Autodesk Inventor part; units mm, degrees
ref_plane "YZ Plane" through (0, 0, 0) normal (1, 0, 0) x (0, 1, 0)
ref_plane "XZ Plane" through (0, 0, 0) normal (0, 1, 0) x (-1, 0, 0)
ref_plane "XY Plane" through (0, 0, 0) normal (0, 0, 1) x (1, 0, 0)
sketch "Sketch1" plane through (0, 0, 0) normal (0, 1, 0) x (-1, 0, 0)
  line L0 (57.5, -173) -> (57.5, -173) construction
  line L1 (-57.5, -173) -> (-57.5, 0) construction
  line L2 (-57.5, 0) -> (57.5, 0)
  line L3 (57.5, 0) -> (57.5, -173) construction
  line L4 (80.5, 0) -> (-80.5, 0) construction
  line L5 (0, -207.6) -> (0, 34.6) construction
  line L6 (57.5, -173) -> (-57.5, -173)
  line L7 (-57.5, -173) -> (-57.5, -173) construction
  line L8 (57.5, 0) -> (-55.1767, 0)
  line L9 (57.5, -40) -> (-57.5, -40) construction
  line L10 (-57.5, -40) -> (-57.5, 0)
  line L11 (-57.5, 0) -> (57.5, 0)
  line L12 (57.5, 0) -> (57.5, -40)
  line L13 (-57.5, -173) -> (-57.5, -40)
  line L14 (57.5, -173) -> (57.5, -40)
  point P0 (0, 0)
  dimension "width" = 115
  dimension "Length" = 173
  dimension "d2" = 115
  dimension "d112" = 40
extrude "Base" add sketch "Sketch1" against normal blind 5
sketch "Sketch11" plane through (0, 0, 0) normal (0, 1, 0) x (1, 0, 0)
  line L0 (0, 207.6) -> (0, -34.6) construction
  line L1 (-57.5, 0) -> (57.5, 0) construction
  line L2 (57.5, 173) -> (-57.5, 173)
  line L3 (-50, 18) -> (50, 18) construction
  line L4 (50, 18) -> (50, 48) construction
  line L5 (50, 48) -> (-50, 48) construction
  line L6 (-50, 48) -> (-50, 18) construction
  point P0 (0, 0)
  point P1 (50, 168)
  point P2 (-50, 168)
  dimension "d91" = 18
  dimension "d92" = 50
  dimension "d93" = 5
  dimension "d94" = 50
  dimension "d113" = 30
hole "Mounting Holes" at (50, 0, -18) at (-50, 0, -18) at (50, 0, -168) at (-50, 0, -168) at (-50, 0, -48) at (50, 0, -48) direction (0, -1, 0) diameter 3.4 depth 6
fillet "Fillet1" radius 5 4 edges at (-57.5, -2.5, 0) (57.5, -2.5, -173) (-57.5, -2.5, -173) (57.5, -2.5, 0)
sketch "Sketch12" plane through (0, 0, 0) normal (0, 1, 0) x (1, 0, 0)
  line L0 (-6, 149) -> (43, 149) construction
  line L1 (43, 149) -> (43, 91) construction
  line L2 (43, 91) -> (-6, 91) construction
  line L3 (-6, 91) -> (-6, 149) construction
  line L4 (-57.5, 168) -> (-57.5, 5)
  line L5 (0, 207.6) -> (0, -34.6)
  line L6 (-52.5, 0) -> (52.5, 0)
  circle A0 centre (-50, 48) radius 1.7
  line L7 (52.5, 173) -> (-52.5, 173)
  circle A1 centre (50, 48) radius 1.7
  circle A2 centre (50, 168) radius 1.7
  point P0 (0, 0)
  point P1 (0, 0)
  point P2 (52.2987, 0)
  point P3 (-57.5, 40)
  point P4 (0, 0)
  dimension "d104" = 58
  dimension "d263" = 24
  dimension "d266" = 49
  dimension "d267" = 7
hole "RasPi Mounting Holes" at (-6, 0, -149) at (43, 0, -149) at (43, 0, -91) at (-6, 0, -91) direction (0, -1, 0) diameter 3.4 depth 6
sketch "Sketch15" plane through (0, 0, 0) normal (0, 1, 0) x (1, 0, 0)
  line L0 (-18, 149) -> (-18, 87.5) construction
  line L1 (-18, 87.5) -> (-50, 87.5) construction
  line L2 (-50, 87.5) -> (-50, 149) construction
  line L3 (-50, 149) -> (-18, 149) construction
  line L4 (-52.5, 0) -> (52.5, 0)
  circle A0 centre (43, 149) radius 1.7
  circle A1 centre (50, 48) radius 1.7
  circle A2 centre (-50, 48) radius 1.7
  point P0 (0, 0)
  point P1 (0, 0)
  dimension "d122" = 32
  dimension "d123" = 61.5
hole "LM2596 Mounting Holes" at (-18, 0, -149) at (-18, 0, -87.5) at (-50, 0, -87.5) at (-50, 0, -149) direction (0, -1, 0) diameter 3.4 depth 6
sketch "Sketch16" plane through (0, 0, 0) normal (0, 1, 0) x (1, 0, 0)
  line L0 (-7.5, 16.5) -> (7.5, 16.5) construction
  line L1 (7.5, 16.5) -> (7.5, 30) construction
  line L2 (7.5, 30) -> (-7.5, 30) construction
  line L3 (-7.5, 30) -> (-7.5, 16.5) construction
  line L4 (52.5, 173) -> (-52.5, 173)
  line L5 (-52.5, 0) -> (52.5, 0)
  point P0 (0, 0)
  point P1 (0, 30)
  point P2 (0, 173)
  dimension "d132" = 15
  dimension "d133" = 13.5
  dimension "d264" = 16.5
hole "Camera Mount Mounting Holes" at (-7.5, 0, -30) at (-7.5, 0, -16.5) at (7.5, 0, -16.5) at (7.5, 0, -30) direction (0, -1, 0) diameter 3.4 depth 6
sketch "Sketch17" plane through (0, 0, 0) normal (0, 1, 0) x (1, 0, 0)
  spline S0 degree 4 poles (20.2958, 49.4851) (20.6789, 48.9084) (23.4396, 47.5095) (25.9197, 47.6138) (27.8901, 48.6422) (29.1867, 50.3145) (29.4114, 52.1793) (28.5047, 55.2295) (25.5201, 55.758) (20.7186, 56.8474) (23.8724, 60.2591) (26.3838, 58.5227) (28.1257, 57.2645) knots 0 0 0 0 0 0.20272 0.281354 0.355201 0.433006 0.519581 0.610324 0.697239 0.780233 1 1 1 1 1
  line L0 (28.1257, 57.2645) -> (29.7111, 59.2874)
  line L1 (20.2958, 49.4851) -> (21.6797, 51.6642)
  spline S1 degree 4 poles (21.6797, 51.6642) (22.294, 51.399) (22.8002, 50.5746) (25.5673, 49.8354) (26.8617, 51.423) (26.2496, 52.8197) (24.0458, 53.1534) (23.329, 53.4897) (21.3928, 54.1292) (20.3004, 55.4262) (19.7305, 56.5103) (20.0555, 59.7919) (23.1279, 61.9518) (27.765, 61.4454) (29.2944, 59.5103) (29.7111, 59.2874) knots 0 0 0 0 0 0.144957 0.205265 0.266901 0.324627 0.385746 0.449033 0.50901 0.575778 0.647334 0.728378 0.816759 1 1 1 1 1
  line L2 (19.0392, 48.0812) -> (19.0392, 61.1238)
  line L3 (19.0392, 61.1238) -> (16.3103, 61.1165)
  line L4 (16.3103, 61.1165) -> (16.3103, 57.2645)
  line L5 (16.3005, 50.6209) -> (16.3005, 54.6823)
  line L6 (16.3005, 54.6823) -> (13.9834, 54.6823)
  line L7 (16.3005, 50.6209) -> (13.9834, 50.6209)
  line L8 (19.0392, 48.0812) -> (13.9055, 48.0812)
  line L9 (16.3103, 57.2645) -> (13.9055, 57.2645)
  spline S2 degree 4 poles (13.9055, 48.0812) (12.4379, 47.8667) (9.7187, 48.6838) (8.9871, 53.4702) (10.0145, 55.7471) (11.812, 57.3277) (13.9055, 57.2645) knots 0 0 0 0 0 0.42418 0.584268 1 1 1 1 1
  spline S3 degree 4 poles (13.9834, 50.6209) (12.498, 50.3895) (10.979, 52.4191) (12.1531, 54.6206) (13.9834, 54.6823) knots 0 0 0 0 0 1 1 1 1 1
  line L10 (5.611, 51.8606) -> (5.611, 61.1378)
  line L11 (5.611, 61.1378) -> (2.2951, 61.1378)
  line L12 (2.2951, 61.1378) -> (2.2951, 60.9623)
  line L13 (2.2951, 60.9623) -> (2.2951, 57.2161)
  line L14 (2.2951, 57.2161) -> (0.5839, 57.2161)
  line L15 (0.5839, 57.2161) -> (-1.936, 61.1378)
  line L16 (-1.936, 61.1378) -> (-5.9376, 61.1378)
  line L17 (-5.9376, 61.1378) -> (-3.4177, 57.2161)
  line L18 (5.611, 51.8606) -> (2.2951, 51.8606)
  line L19 (2.2951, 51.8606) -> (2.2951, 53.8306)
  line L20 (2.2951, 53.8306) -> (-1.6405, 53.8306)
  line L21 (-1.6405, 53.8306) -> (-1.6405, 51.2415)
  line L22 (-1.6405, 51.2415) -> (5.611, 51.2415)
  line L23 (5.611, 51.2415) -> (5.611, 47.9336)
  line L24 (5.611, 47.9336) -> (-3.7057, 47.9336)
  line L25 (-5.0121, 49.3829) -> (-5.0121, 55.5531)
  arc A0 (-3.4177, 57.2161) -> (-5.0121, 55.5531) centre (-3.281, 55.4892) ccw
  arc A1 (-5.0121, 49.3829) -> (-3.7057, 47.9336) centre (-2.6718, 50.1788) ccw
  line L26 (-6.9039, 47.9336) -> (-10.2687, 47.9336)
  line L27 (-10.2687, 47.9336) -> (-10.2687, 61.1378)
  line L28 (-10.2687, 61.1378) -> (-6.9039, 61.1378)
  line L29 (-6.9039, 61.1378) -> (-6.9039, 47.9336)
  line L30 (-11.8026, 47.9336) -> (-11.8026, 51.2415)
  line L31 (-11.8026, 51.2415) -> (-15.1713, 51.2415)
  line L32 (-15.1713, 51.2415) -> (-15.1713, 61.1378)
  line L33 (-15.1713, 61.1378) -> (-18.4823, 61.1378)
  line L34 (-18.4823, 61.1378) -> (-18.4823, 47.9336)
  line L35 (-18.4823, 47.9336) -> (-11.8026, 47.9336)
  line L36 (-19.0962, 47.9336) -> (-19.0962, 51.2415)
  line L37 (-19.0962, 51.2415) -> (-21.5406, 51.2415)
  line L38 (-21.5406, 51.2415) -> (-23.787, 47.9336)
  line L39 (-23.787, 47.9336) -> (-19.0962, 47.9336)
  line L40 (-24.4617, 47.9274) -> (-24.4617, 61.1378)
  line L41 (-24.4617, 61.1378) -> (-27.7836, 61.1378)
  line L42 (-27.7836, 61.1378) -> (-27.7836, 47.9274)
  line L43 (-27.7836, 47.9274) -> (-24.4617, 47.9274)
  line L44 (-28.3589, 52.8456) -> (-28.3589, 56.1975)
  line L45 (-28.3589, 56.1975) -> (-30.851, 56.1975)
  line L46 (-30.851, 52.8456) -> (-28.3589, 52.8456)
  line L47 (-27.7836, 47.9274) -> (-27.7836, 51.2654)
  line L48 (-27.7836, 51.2654) -> (-32.8922, 51.2654)
  line L49 (-32.8922, 47.9274) -> (-27.7836, 47.9274)
  line L50 (-32.8922, 47.9274) -> (-35.0606, 51.2654)
  line L51 (-35.0606, 51.2654) -> (-32.8922, 51.2654)
  line L52 (-30.851, 52.8456) -> (-33.0635, 52.8734)
  line L53 (-33.0635, 52.8734) -> (-30.851, 56.1975)
  line L54 (-27.7836, 57.7985) -> (-35.0607, 57.7985)
  line L55 (-35.0607, 57.7985) -> (-32.8922, 61.1378)
  line L56 (-32.8922, 61.1378) -> (-27.7836, 61.1378)
  point P0 (21.8312, 48.4826)
  point P1 (24.6762, 47.7793)
  point P2 (27.8239, 48.7935)
  point P3 (29.2122, 52.0376)
  point P4 (25.048, 55.8974)
  point P5 (22.697, 57.0989)
  point P6 (22.9251, 58.2765)
  point P7 (24.696, 58.9116)
  point P8 (28.2025, 54.5741)
  point P9 (28.8947, 50.19)
  point P10 (26.5311, 48.0478)
  point P11 (22.4682, 51.1588)
  point P12 (23.9337, 50.486)
  point P13 (25.8462, 50.5785)
  point P14 (26.5371, 51.481)
  point P15 (26.0534, 52.5205)
  point P16 (24.2764, 53.1685)
  point P17 (23.1794, 53.5189)
  point P18 (21.5574, 54.2619)
  point P19 (20.447, 55.336)
  point P20 (19.9671, 56.4765)
  point P21 (20.2871, 59.0572)
  point P22 (22.4689, 61.0346)
  point P23 (26.4542, 61.1331)
  point P24 (29.0183, 59.8364)
  point P25 (11.4211, 48.5559)
  point P26 (9.78, 50.5097)
  point P27 (9.4515, 53.0365)
  point P28 (9.8728, 54.8339)
  point P29 (11.0323, 56.3265)
  point P30 (12.7057, 51.0411)
  point P31 (12.0375, 52.3737)
  point P32 (12.4422, 53.8787)
  point P33 (-27.7836, 51.2654)
  point P34 (-3.281, 55.4892)
extrude "SP RITE Logo" [suppressed]
equation "\"d2\" = width"
equation "\"d95\" = HoleDia"
equation "\"d105\" = HoleDia"
equation "\"d125\" = HoleDia"
equation "\"d135\" = HoleDia"
equation "\"HoleDia\" = 3.4"
properties part number "top plate"
Could you check a few things on this model? Use its own coordinates, in mm. Give positions to 0.01 mm unless a question says otherwise; leave off trailing zeros. Order: outer loops, then holes, each group sorted by start corner. A loop starts at its lowest first (then second) coordinate and runs counter-clockwise, first axis right, second up.
Item 1: I'm going to push a flat-ended pin straight in: pin 1 (2 mm diameter, centred on x = -6, z = -91, fed in from -Y). Where does the tip first touch, or does it pass through?
Item 2: If we section it at C-C, the plane x = -18: Write out the boundary of the cut face in (y, z), plus the area to 3 significant figures.
Item 3: I need wall thicknesses on line 1 (Z direction, x = -50, y = -2.7); line 2 (X direction, y = -1.1, z = -48); line 3 (Z direction, x = 7.5, y = -3.9). Which ranges of each line are inside material? Lowest first, please.
Item 4: If we section it at A-A, the plane z = -48: Write out the boundary of the cut face in (x, y).
Item 5: If we mould it in two halves opening along X, with no side actions, what happens to faces 1 (the face through (56, -2.54, -171.57)), 2 (the face through (51.03, -2.54, -49.35)), 3 (the face through (-56.07, -2.54, -171.5))? For each: pulls with the +X half, pulls with the -X half, needs draft (parallel to the pull), parting line crosses it, or undercut.
Item 6: If we section it at B-B, the plane x = -50: Write out the boundary of the cut face in (y, z), plus the area to 3 significant figures.
Values:
1. pin 1: passes through
2. outline: (-5, -173) - (0, -173) - (0, -150.7) - (-5, -150.7) - close; (-5, -147.3) - (0, -147.3) - (0, -89.2) - (-5, -89.2) - close; (-5, -85.8) - (0, -85.8) - (0, 0) - (-5, 0) - close
2. area: 831 mm2
3. line 1: z = -173 to -169.7, -166.3 to -150.7, -147.3 to -89.2, -85.8 to -49.7, -46.3 to -19.7, -16.3 to 0
3. line 2: x = -57.5 to -51.7, -48.3 to 48.3, 51.7 to 57.5
3. line 3: z = -173 to -31.7, -28.3 to -18.2, -14.8 to 0
4. outline: (-57.5, -5) - (-51.7, -5) - (-51.7, 0) - (-57.5, 0) - close; (-48.3, -5) - (48.3, -5) - (48.3, 0) - (-48.3, 0) - close; (51.7, -5) - (57.5, -5) - (57.5, 0) - (51.7, 0) - close
5. face 1: pulls with the +X half
5. face 2: undercut
5. face 3: pulls with the -X half
6. outline: (-5, -173) - (0, -173) - (0, -169.7) - (-5, -169.7) - close; (-5, -166.3) - (0, -166.3) - (0, -150.7) - (-5, -150.7) - close; (-5, -147.3) - (0, -147.3) - (0, -89.2) - (-5, -89.2) - close; (-5, -85.8) - (0, -85.8) - (0, -49.7) - (-5, -49.7) - close; (-5, -46.3) - (0, -46.3) - (0, -19.7) - (-5, -19.7) - close; (-5, -16.3) - (0, -16.3) - (0, 0) - (-5, 0) - close
6. area: 780 mm2
